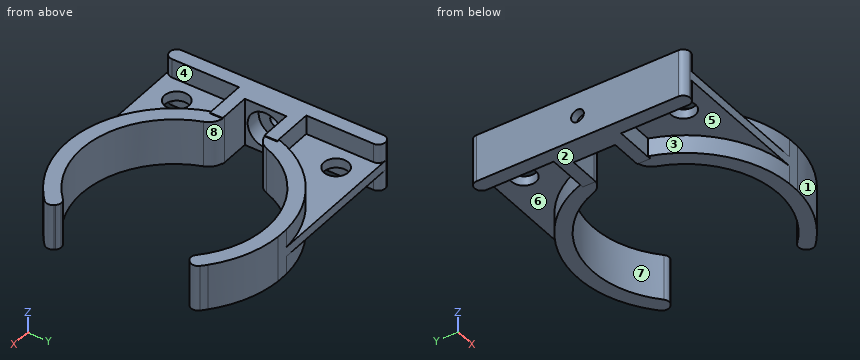
from build123d import *

# Parameters (mm, degrees)
F1_DEPTH  = 7.5
F2_W      = 21.2
F2_H      = 15
F3_DEPTH  = 5.45
F4_W      = 4.05
F4_H      = 15
F5_DEPTH  = 10
F6_R      = 3.85
F7_DEPTH  = 1.5
F8_DEPTH  = 7.25
F9_R      = 5
F10_R     = 5.65
F11_DEPTH = 5
F12_R     = 2
F13_DEPTH = 25


with BuildPart() as f1:
    # F0 (on Top) → F1 (new body, symmetric)
    with BuildSketch(Plane.XY):
        with BuildLine():
            ThreePointArc((2.25, 31.755662), (1.607293, 33.307293), (0.055662, 33.95))
            Line((0.055662, 33.95), (-0.055662, 33.95))
            ThreePointArc((-0.055662, 33.95), (-1.607293, 33.307293), (-2.25, 31.755662))
            Line((-2.25, 31.755662), (-2.25, -31.755662))
            ThreePointArc((-2.25, -31.755662), (-1.607293, -33.307293), (-0.055662, -33.95))
            Line((-0.055662, -33.95), (0.055662, -33.95))
            ThreePointArc((0.055662, -33.95), (1.607293, -33.307293), (2.25, -31.755662))
            Line((2.25, -31.755662), (2.25, 31.755662))
        make_face()
    extrude(amount=F1_DEPTH, both=True)

    # F2 (on Right) → F3 (join)
    with BuildSketch(Plane.YZ):
        Rectangle(F2_W, F2_H)
    extrude(amount=F3_DEPTH)

    # F4 (on face) → F5 (join)
    with BuildSketch(Plane.YZ.offset(5.45)):
        with Locations((8.575, 0)):
            Rectangle(F4_W, F4_H)
        with Locations((-8.575, 0)):
            Rectangle(F4_W, F4_H)
    extrude(amount=F5_DEPTH)

    # F6 (on Top) → F7 (join, symmetric)
    with BuildSketch(Plane.XY):
        with BuildLine():
            Line((44.995906, 33.95), (0.055662, 33.95))
            ThreePointArc((0.055662, 33.95), (1.607293, 33.307293), (2.25, 31.755662))
            Line((2.25, 31.755662), (2.25, 10.6))
            Line((2.25, 10.6), (14.533719, 10.6))
            ThreePointArc((14.533719, 10.6), (26.154887, 26.984474), (44.995906, 33.95))
        make_face()
        with Locations((9.6, 25.1)):
            Circle(F6_R, mode=Mode.SUBTRACT)
        with BuildLine():
            Line((2.25, -10.6), (2.25, -31.755662))
            ThreePointArc((2.25, -31.755662), (1.607293, -33.307293), (0.055662, -33.95))
            Line((0.055662, -33.95), (44.995906, -33.95))
            ThreePointArc((44.995906, -33.95), (26.154887, -26.984474), (14.533719, -10.6))
            Line((14.533719, -10.6), (2.25, -10.6))
        make_face()
        with Locations((9.6, -25.1)):
            Circle(F6_R, mode=Mode.SUBTRACT)
    extrude(amount=F7_DEPTH, both=True)

    # F6 (on Top) → F8 (join, symmetric)
    with BuildSketch(Plane.XY):
        with BuildLine():
            Line((48.682367, 33.95), (44.995906, 33.95))
            ThreePointArc((44.995906, 33.95), (26.154887, 26.984474), (14.533719, 10.6))
            Line((14.533719, 10.6), (15.45, 10.6))
            Line((15.45, 10.6), (15.45, 6.55))
            Line((15.45, 6.55), (18.331945, 6.55))
            ThreePointArc((18.331945, 6.55), (38.555461, 28.052508), (67.215495, 20.984912))
            ThreePointArc((67.215495, 20.984912), (67.968637, 20.506465), (68.85, 20.367419))
            Line((68.85, 20.367419), (68.85, 25.913739))
            ThreePointArc((68.85, 25.913739), (59.424836, 31.584809), (48.682367, 33.95))
        make_face()
        with BuildLine():
            Line((15.45, -10.6), (14.533719, -10.6))
            ThreePointArc((14.533719, -10.6), (26.154887, -26.984474), (44.995906, -33.95))
            Line((44.995906, -33.95), (48.682367, -33.95))
            ThreePointArc((48.682367, -33.95), (59.424836, -31.584809), (68.85, -25.913739))
            Line((68.85, -25.913739), (68.85, -20.367419))
            ThreePointArc((68.85, -20.367419), (67.968637, -20.506465), (67.215495, -20.984912))
            ThreePointArc((67.215495, -20.984912), (38.555461, -28.052508), (18.331945, -6.55))
            Line((18.331945, -6.55), (15.45, -6.55))
            Line((15.45, -6.55), (15.45, -10.6))
        make_face()
        with BuildLine():
            ThreePointArc((70.503742, 24.412834), (69.689198, 25.176869), (68.85, 25.913739))
            Line((68.85, 25.913739), (68.85, 20.367419))
            ThreePointArc((68.85, 20.367419), (69.721282, 20.594438), (70.428051, 21.152243))
            Line((70.428051, 21.152243), (70.660364, 21.430287))
            ThreePointArc((70.660364, 21.430287), (71.167762, 22.952317), (70.503742, 24.412834))
        make_face()
        with BuildLine():
            Line((68.85, -20.367419), (68.85, -25.913739))
            ThreePointArc((68.85, -25.913739), (69.689198, -25.176869), (70.503742, -24.412834))
            ThreePointArc((70.503742, -24.412834), (71.167762, -22.952317), (70.660364, -21.430287))
            Line((70.660364, -21.430287), (70.428051, -21.152243))
            ThreePointArc((70.428051, -21.152243), (69.721282, -20.594438), (68.85, -20.367419))
        make_face()
    extrude(amount=F8_DEPTH, both=True)

    # F9
    f9_edges = [f1.edges().sort_by_distance(p)[0] for p in [
        (18.331945, 6.55, 0),
        (18.331945, -6.55, 0),
    ]]
    fillet(f9_edges, radius=F9_R)

    # F10 (on face) → F11 (cut)
    with BuildSketch(Plane.YZ.offset(5.45)):
        Circle(F10_R)
    extrude(amount=-F11_DEPTH, mode=Mode.SUBTRACT)

    # F12 (on face) → F13 (cut)
    with BuildSketch(Plane.YZ.offset(0.45)):
        Circle(F12_R)
    extrude(amount=-F13_DEPTH, mode=Mode.SUBTRACT)


solid = f1.part
Here's how the part is built. I have some questions about the finished solid (model axes, mm). Face numbers are marked on the shaded views. A direction names the side the tool comes from. Round coordinates to 2 decimals unless told otherwise and drop trailing zeros. Loops run counter-clockwise (first coordinate to the right, second up) from the corner with the lowest first, then second, coordinate; pieces in that order, holes last.
1. We'd pull the mould along X, two halves only. Please class the marked faces 1, 2 and 3: +X half, -X half, draft (parallel to the pull), parting line (faces both ways), or undercut.
Answer list:
face 1: +X half
face 2: draft
face 3: undercut
2. If we section it at B-B on y = 0: Write out the boundary of the cut face in (x, z).
Answer list:
outline: (-2.25, -7.5) - (5.45, -7.5) - (5.45, -5.65) - (0.45, -5.65) - (0.45, -2) - (-2.25, -2) - close; (-2.25, 2) - (0.45, 2) - (0.45, 5.65) - (5.45, 5.65) - (5.45, 7.5) - (-2.25, 7.5) - close
3. Which directions (+Z, -Z, +X, -X, +Y, -Y) give clear straight access to the entire face, cutting with the end or side of a thin tool? Please do the marked faces 4, 5, 6, 7 and 8.
Answer list:
face 4: +Z, -Y
face 5: -Z, -Y
face 6: -Z, +Y
face 7: +Z, -Z
face 8: +Z, -Z, +X
4. If I drill on line 1 along Z through (x, y) = (-1.35, 0); line 2 along Y through (x, z) = (9.6, -0.5); line 3 along Z through (x, y) = (5, 0), over which ranges is the centre line in solid material (lowest first)?
Answer list:
line 1: z = -7.5 to -2, 2 to 7.5
line 2: y = -33.95 to -28.95, -21.25 to -6.55, 6.55 to 21.25, 28.95 to 33.95
line 3: z = -7.5 to -5.65, 5.65 to 7.5
5. If we section it at A-A on z = 0: Count the separate pieces of the cut face and the enclosed holes in it, plus the area to 3 significant figures.
Answer list:
separate pieces: 2
enclosed holes: 2
area: 1,910 mm2
6. If we section it at C-C on x = 9.6: Write out the boundary of the cut face in (y, z), plus the area to 3 significant figures.
Answer list:
outline: (-33.95, -1.5) - (-28.95, -1.5) - (-28.95, 1.5) - (-33.95, 1.5) - close; (-21.25, -1.5) - (-10.6, -1.5) - (-10.6, -7.5) - (-6.55, -7.5) - (-6.55, 7.5) - (-10.6, 7.5) - (-10.6, 1.5) - (-21.25, 1.5) - close; (6.55, -7.5) - (10.6, -7.5) - (10.6, -1.5) - (21.25, -1.5) - (21.25, 1.5) - (10.6, 1.5) - (10.6, 7.5) - (6.55, 7.5) - close; (28.95, -1.5) - (33.95, -1.5) - (33.95, 1.5) - (28.95, 1.5) - close
area: 215 mm2
7. For P1, Ø3, axis at y = 18.5, z = 4.5, coming from the +X side; P2, Ø1.8, axis at x = 5.5, z = -4, coming from the -Y side; P3, Ø1.5, axis at x = 59.5, z = 0, coming from the +Y side, each with a flat end and sliding along its axis, tell me the tip position at first contact or that it passes through.
Answer list:
P1: stops at x = 25.5
P2: stops at y = -10.6
P3: stops at y = 31.85
8. If we section it at D-D on x = 56: Write out the boundary of the cut face in (y, z).
Answer list:
outline: (-32.74, -7.25) - (-27.78, -7.25) - (-27.78, 7.25) - (-32.74, 7.25) - close; (27.78, -7.25) - (32.74, -7.25) - (32.74, 7.25) - (27.78, 7.25) - close
